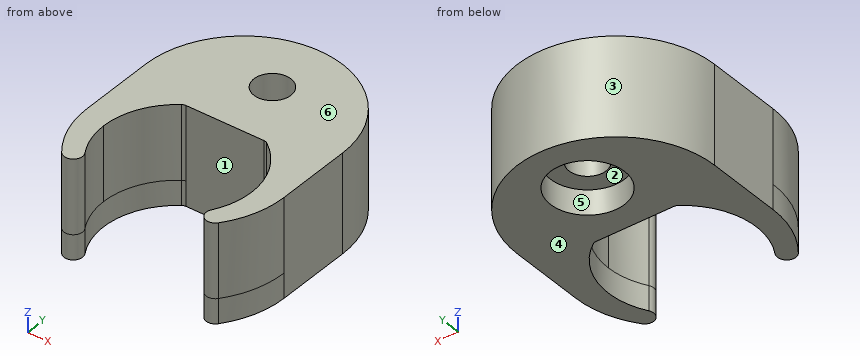
Autodesk Inventor part; units mm, degrees
ref_plane "Work Plane1" through (127.525, 15.075, -31.525) normal (0, 0, -1) x (-1, 0, 0)
ref_plane "YZ Plane" through (0, 0, 0) normal (1, 0, 0) x (0, 1, 0)
ref_plane "XZ Plane" through (0, 0, 0) normal (0, 1, 0) x (-1, 0, 0)
sketch "Sketch1" plane through (0, 0, 0) normal (0, 0, 1) x (1, 0, 0)
  line L0 (127.525, 5) -> (129.95, 5)
  line L1 (127.525, 15.075) -> (127.525, 5)
  line L2 (115.375, 15.075) -> (127.525, 15.075)
  line L3 (115.375, 5) -> (115.375, 15.075)
  line L4 (112.95, 5) -> (115.375, 5)
  line L5 (129.95, 5) -> (129.95, 25.025)
  line L6 (115.45, 10) -> (115.45, 6)
  arc A0 (115.45, 10) -> (118.000243, 5.090909) centre (121.45, 10) ccw
  arc A1 (118.000243, 5.090909) -> (118.287722, 5) centre (118.287722, 5.5) ccw
  line L7 (116.45, 5) -> (118.287722, 5)
  arc A2 (115.45, 6) -> (116.45, 5) centre (116.45, 6) ccw
  line L8 (118.287722, 15) -> (116.45, 15)
  arc A3 (118.287722, 15) -> (118.000243, 14.909091) centre (118.287722, 14.5) ccw
  arc A4 (118.000243, 14.909091) -> (115.45, 10) centre (121.45, 10) ccw
  line L9 (115.45, 14) -> (115.45, 10)
  arc A5 (116.45, 15) -> (115.45, 14) centre (116.45, 14) ccw
  line L10 (127.45, 10) -> (127.45, 14)
  arc A6 (127.45, 10) -> (124.899757, 14.909091) centre (121.45, 10) ccw
  arc A7 (124.899757, 14.909091) -> (124.612278, 15) centre (124.612278, 14.5) ccw
  line L11 (126.45, 15) -> (124.612278, 15)
  arc A8 (127.45, 14) -> (126.45, 15) centre (126.45, 14) ccw
  line L12 (124.612278, 5) -> (126.45, 5)
  arc A9 (124.612278, 5) -> (124.899757, 5.090909) centre (124.612278, 5.5) ccw
  arc A10 (124.899757, 5.090909) -> (127.45, 10) centre (121.45, 10) ccw
  line L13 (127.45, 6) -> (127.45, 10)
  arc A11 (126.45, 5) -> (127.45, 6) centre (126.45, 6) ccw
  arc A12 (118.000243, 5.090909) -> (118.287722, 5) centre (118.287722, 5.5) ccw
  arc A13 (118.000243, 14.909091) -> (118.000243, 5.090909) centre (121.45, 10) ccw
  arc A14 (118.287722, 15) -> (118.000243, 14.909091) centre (118.287722, 14.5) ccw
  line L14 (118.287722, 15) -> (124.612278, 15)
  arc A15 (124.899757, 14.909091) -> (124.612278, 15) centre (124.612278, 14.5) ccw
  arc A16 (124.899757, 5.090909) -> (124.899757, 14.909091) centre (121.45, 10) ccw
  arc A17 (124.612278, 5) -> (124.899757, 5.090909) centre (124.612278, 5.5) ccw
  line L15 (124.612278, 5) -> (118.287722, 5)
  line L16 (127.45, 15.075) -> (129.45, 15.075)
  line L17 (129.45, 15.075) -> (129.45, 5)
  line L18 (129.45, 5) -> (127.45, 5)
  line L19 (127.45, 5) -> (127.45, 15.075)
  line L20 (121.45, 10) -> (121.45, 5)
  arc A18 (127.157107, 5.292893) -> (129.45, 10.828427) centre (121.621573, 10.828427) ccw
  line L21 (115.45, 15.075) -> (113.45, 15.075)
  line L22 (113.45, 15.075) -> (113.45, 5)
  line L23 (113.45, 5) -> (115.45, 5)
  line L24 (115.45, 5) -> (115.45, 15.075)
  arc A19 (113.45, 10.828427) -> (115.742893, 5.292893) centre (121.278427, 10.828427) ccw
  line L25 (121.45, 25) -> (121.45, 15)
  circle A20 centre (121.45, 20) radius 1.5
  circle A21 centre (121.45, 20) radius 3
  line L26 (129.45, 15) -> (113.45, 15)
  line L27 (113.45, 15) -> (113.45, 25)
  line L28 (113.45, 25) -> (129.45, 25)
  line L29 (129.45, 25) -> (129.45, 15)
  arc A22 (129.45, 17) -> (121.45, 25) centre (121.45, 17) ccw
  arc A23 (121.45, 25) -> (113.45, 17) centre (121.45, 17) ccw
  circle A24 centre (121.45, 20) radius 1.4375
  line L30 (129.95, 25.025) -> (112.95, 25.025)
  line L31 (112.95, 25.025) -> (112.95, 5)
  point P0 (0, 0)
  point P1 (112.95, 16.464466)
  point P2 (115.742893, 5.292893)
  point P3 (127.45, 5.602175)
  point P4 (115.45, 5.602175)
  point P5 (115.45, 15)
  point P6 (127.45, 15)
  dimension "d0" = 2
  dimension "d2" = 3
  dimension "d3" = 6
  dimension "d10" = 10
ref_plane "Work Plane1" through (127.525, 15.075, -31.525) normal (0, 0, -1) x (-1, 0, 0)
sketch "Sketch1 outline for Extrusion1" plane through (0, 0, 0) normal (0, 0, 1) x (1, 0, 0)
  arc A0 (124.612278, 15) -> (124.899757, 14.909091) centre (124.612278, 14.5) cw
  line L0 (118.287722, 15) -> (124.612278, 15)
  arc A1 (124.899757, 14.909091) -> (127.45, 10) centre (121.45, 10) cw
  arc A2 (118.000243, 14.909091) -> (118.287722, 15) centre (118.287722, 14.5) cw
  arc A3 (127.45, 10) -> (124.899757, 5.090909) centre (121.45, 10) cw
  arc A4 (115.45, 10) -> (118.000243, 14.909091) centre (121.45, 10) cw
  arc A5 (124.899757, 5.090909) -> (124.612278, 5) centre (124.612278, 5.5) cw
  arc A6 (118.000243, 5.090909) -> (115.45, 10) centre (121.45, 10) cw
  line L1 (124.612278, 5) -> (126.45, 5)
  arc A7 (118.287722, 5) -> (118.000243, 5.090909) centre (118.287722, 5.5) cw
  arc A8 (126.45, 5) -> (127.157107, 5.292893) centre (126.45, 6) ccw
  line L2 (116.45, 5) -> (118.287722, 5)
  arc A9 (127.157107, 5.292893) -> (129.45, 10.828427) centre (121.621573, 10.828427) ccw
  arc A10 (115.742893, 5.292893) -> (116.45, 5) centre (116.45, 6) ccw
  line L3 (129.45, 10.828427) -> (129.45, 15.075)
  arc A11 (113.45, 10.828427) -> (115.742893, 5.292893) centre (121.278427, 10.828427) ccw
  line L4 (129.45, 15.075) -> (129.45, 17)
  line L5 (113.45, 15.075) -> (113.45, 10.828427)
  arc A12 (129.45, 17) -> (121.45, 25) centre (121.45, 17) ccw
  line L6 (113.45, 17) -> (113.45, 15.075)
  arc A13 (121.45, 25) -> (113.45, 17) centre (121.45, 17) ccw
  circle A14 centre (121.45, 20) radius 1.5
extrude "Extrusion1" add sketch "Sketch1 outline for Extrusion1" against normal blind 6 from surface at -31.525
fillet "Fillet1" radius 0.75 4 edges at (124.8998, 5.0909, -34.525) (118.0002, 5.0909, -34.525) (124.6123, 5, -34.525) (118.2877, 5, -34.525)
sketch "Sketch2" plane through (121.45, 14.820968, -37.525) normal (0, 0, -1) x (-1, 0, 0)
  arc A0 (6.362384, -8.784005) -> (8, -3.992541) centre (0.171573, -3.992541) ccw
  line L0 (8, 2.179032) -> (8, -3.992541)
  line L1 (-8, -3.992541) -> (-8, 2.179032)
  arc A1 (-8, -3.992541) -> (-6.362384, -8.784005) centre (-0.171573, -3.992541) ccw
  arc A2 (-3.449757, 0.088123) -> (-5.128245, -7.935627) centre (0, -4.820968) ccw
  arc A3 (-3.162278, 0.179032) -> (-3.449757, 0.088123) centre (-3.162278, -0.320968) ccw
  arc A4 (3.449757, 0.088123) -> (3.162278, 0.179032) centre (3.162278, -0.320968) ccw
  arc A5 (5.128245, -7.935627) -> (3.449757, 0.088123) centre (0, -4.820968) ccw
  circle A6 centre (0, 5.179032) radius 3
  line L2 (3.162278, 0.179032) -> (-3.162278, 0.179032)
  circle A7 centre (0, 5.179032) radius 1.5
  arc A8 (8, 2.179032) -> (-8, 2.179032) centre (0, 2.179032) ccw
  arc A9 (5.128245, -7.935627) -> (6.362384, -8.784005) centre (5.769275, -8.32496) ccw
  arc A10 (-6.362384, -8.784005) -> (-5.128245, -7.935627) centre (-5.769275, -8.32496) ccw
  point P0 (121.45, -14.820968)
  dimension "d7" = 6
sketch "Sketch2 outline for Extrusion2" plane through (121.45, 14.820968, -37.525) normal (0, 0, -1) x (-1, 0, 0)
  arc A0 (5.128245, -7.935627) -> (6.362384, -8.784005) centre (5.769275, -8.32496) ccw
  arc A1 (3.449757, 0.088123) -> (5.128245, -7.935627) centre (0, -4.820968) cw
  arc A2 (6.362384, -8.784005) -> (8, -3.992541) centre (0.171573, -3.992541) ccw
  arc A3 (3.162278, 0.179032) -> (3.449757, 0.088123) centre (3.162278, -0.320968) cw
  line L0 (8, -3.992541) -> (8, 2.179032)
  line L1 (-3.162278, 0.179032) -> (3.162278, 0.179032)
  arc A4 (8, 2.179032) -> (-8, 2.179032) centre (0, 2.179032) ccw
  arc A5 (-3.449757, 0.088123) -> (-3.162278, 0.179032) centre (-3.162278, -0.320968) cw
  line L2 (-8, 2.179032) -> (-8, -3.992541)
  arc A6 (-5.128245, -7.935627) -> (-3.449757, 0.088123) centre (0, -4.820968) cw
  arc A7 (-8, -3.992541) -> (-6.362384, -8.784005) centre (-0.171573, -3.992541) ccw
  arc A8 (-6.362384, -8.784005) -> (-5.128245, -7.935627) centre (-5.769275, -8.32496) ccw
  circle A9 centre (0, 5.179032) radius 3
extrude "Extrusion2" add sketch "Sketch2 outline for Extrusion2" along normal blind 2
properties part number "Y Stage Motor Clamp V5"
Read the model definition and answer for the solid it produces. Units are mm, in the model's axes. Face numbers are marked on the shaded views. A direction names the side the tool comes from. Give positions to 0.01 mm unless a question says otherwise; leave off trailing zeros. Write each loop counter-clockwise with the first axis right and the second up, starting at its lowest first coordinate (ties: lowest second). Pieces come first, ordered by that corner, then holes. Notation, with made-up numbers: (46, -32.5) -> (97, -32.5) arc R6 ccw to (97, -22.5) -> close; hole circle Ø4 at (4, 7.5). An arc over 180 degrees is marked (long way). Answer as a JSON object with one key per item and string values. Group by question number.
1) Find section C-C (y = 11.5). Write down the section's boundary in (x, z) (3 decimals).
2) Each of these flat-tipped pins is pushed along its axis until it touches: P1, Ø1.9, axis at x = 122, z = -34, coming from the -Y side; P2, Ø4, axis at x = 117, z = -33.5, coming from the +Y side; P3, Ø3, axis at x = 122, y = 20.5, coming from the -Z side (3 decimals); P4, Ø1.8, axis at x = 121.45, y = 20, coming from the -Z side. Where does it stop, or does it pass through?
3) Consider L1, parallel to Y at x = 121.45, z = -38.4; L2, parallel to Y at x = 121.45, z = -35.5; L3, parallel to X at y = 19.25, z = -34. Determine where each line is inside the solid, lowest interval first. Write a range as from..to.
4) Find section B-B (y = 20). Write down the section's boundary in (x, z) (3 decimals), and give its area (3 significant figures).
5) Find section A-A (x = 121.45). Write down the section's boundary in (y, z) (3 decimals), and give its area (3 significant figures).
6) Find section D-D (x = 126.25). Write down the section's boundary in (y, z) (3 decimals).
7) The mould has two halves that part along Z. Classify the marked faces 4, 5 and 6: +Z half, -Z half, draft (parallel to the pull), parting line (faces both ways), or undercut.
8) A tool of negligible diameter and unlimited length cuts with its end or side. For the marked faces 1, 2 and 3, from which of +Z, -Z, +X, -X, +Y, -Y can it reach the whole face along a straight path? Write none if from no direction.
Values follow:
{
 "1": {"outline": "(113.45, -39.525) -> (115.641, -39.525) -> (115.641, -31.525) -> (113.45, -31.525) -> close; (127.259, -39.525) -> (129.45, -39.525) -> (129.45, -31.525) -> (127.259, -31.525) -> close"},
 "2": {"P1": "stops at y = 15", "P2": "stops at y = 24.62", "P3": "stops at z = -37.525", "P4": "passes through"},
 "3": {"L1": "y = 15..17, 23..25", "L2": "y = 15..18.5, 21.5..25", "L3": "x = 113.77..120.15, 122.75..129.13"},
 "4": {"outline": "(114.034, -39.525) -> (118.45, -39.525) -> (118.45, -37.525) -> (119.95, -37.525) -> (119.95, -31.525) -> (114.034, -31.525) -> close; (122.95, -37.525) -> (124.45, -37.525) -> (124.45, -39.525) -> (128.866, -39.525) -> (128.866, -31.525) -> (122.95, -31.525) -> close", "area": "88.7 mm2"},
 "5": {"outline": "(15, -39.525) -> (17, -39.525) -> (17, -37.525) -> (18.5, -37.525) -> (18.5, -31.525) -> (15, -31.525) -> close; (21.5, -37.525) -> (23, -37.525) -> (23, -39.525) -> (25, -39.525) -> (25, -31.525) -> (21.5, -31.525) -> close", "area": "50.0 mm2"},
 "6": {"outline": "(13.6, -39.525) -> (23.4, -39.525) -> (23.4, -31.525) -> (13.6, -31.525) -> close"},
 "7": {"face 4": "-Z half", "face 5": "draft", "face 6": "+Z half"},
 "8": {"face 1": "+Z, -Z, -Y", "face 2": "-Z", "face 3": "+Z, -Z, +Y"}
}
